For this review, use the dimensioned drawing (mm, ordinates from the lowest corner) and the shaded views. A direction names the side the tool comes from. Give positions to 0.01 mm unless a question says otherwise; leave off trailing zeros. Order: outer loops, then holes, each group sorted by start corner. A loop starts at its lowest first (then second) coordinate and runs counter-clockwise, first axis right, second up. Notation, with made-up numbers: (71.25, -9.5) - (106.25, -9.5) arc R15 ccw to (106.25, 16.5) - close; hole circle Ø8 at (60.5, 21). An arc over 180 degrees is marked (long way). One line per item, written item: value.
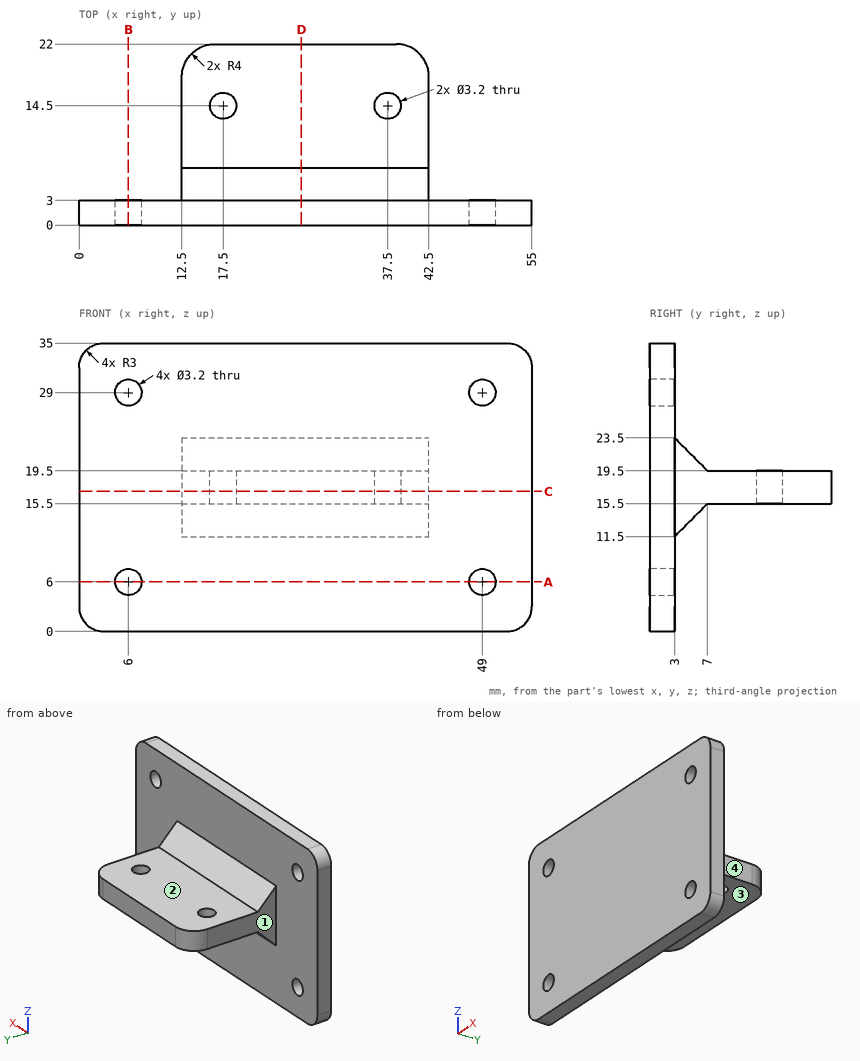
(1) Wall thickness on line 1 (X direction, y = 2.3, z = 29); line 2 (Y direction, x = 17.5, z = 18.65); line 3 (Y direction, x = 5, z = 17.5): over which ranges is each line inside the solid? List them lowest first. Write a range as from..to.
Answers below:
line 1: x = 0..4.4, 7.6..47.4, 50.6..55
line 2: y = 0..12.9, 16.1..22
line 3: y = 0..3
(2) Take a section at B-B (x = 6). Write out the cut boundary in (y, z).
Answers below:
outline: (0, 0) - (3, 0) - (3, 4.4) - (0, 4.4) - close; (0, 7.6) - (3, 7.6) - (3, 27.4) - (0, 27.4) - close; (0, 30.6) - (3, 30.6) - (3, 35) - (0, 35) - close
(3) Machinability: for the marked faces 1, 2, 3 and 4, which of the approach directions +Z, -Z, +X, -X, +Y, -Y give a long, thin tool a straight path to every point of the face, cutting with its end or side? Answer none if there is none.
Answers below:
face 1: +Z, -Z, -X, +Y
face 2: +Z, +X, -X, +Y
face 3: -Z, +X, -X, +Y
face 4: +Z, -Z, +X, +Y
(4) Take a section at A-A (z = 6). Write out the cut boundary in (x, y), then the cut area to 3 significant figures.
Answers below:
outline: (0, 0) - (4.4, 0) - (4.4, 3) - (0, 3) - close; (7.6, 0) - (47.4, 0) - (47.4, 3) - (7.6, 3) - close; (50.6, 0) - (55, 0) - (55, 3) - (50.6, 3) - close
area: 146 mm^2
(5) Take a section at C-C (z = 17). Write out the cut boundary in (x, y), then the cut area to 3 significant figures.
Answers below:
outline: (0, 0) - (55, 0) - (55, 3) - (42.5, 3) - (42.5, 18) arc R4 ccw to (38.5, 22) - (16.5, 22) arc R4 ccw to (12.5, 18) - (12.5, 3) - (0, 3) - close; hole circle Ø3.2 at (17.5, 14.5); hole circle Ø3.2 at (37.5, 14.5)
area: 712 mm^2
(6) For P1, Ø5, axis at x = 37.5, y = 14.5, coming from the -Z side; P2, Ø6, axis at x = 20, y = 11, coming from the +Z side; P3, Ø9.5, axis at y = 9, z = 16.5, coming from the -X side, all flat-tipped, find the tip position at first contact; note any pin that passes through.
Answers below:
P1: stops at z = 15.5
P2: stops at z = 19.5
P3: stops at x = 12.5
(7) Take a section at D-D (x = 27). Write out the cut boundary in (y, z).
Answers below:
outline: (0, 0) - (3, 0) - (3, 11.5) - (7, 15.5) - (22, 15.5) - (22, 19.5) - (7, 19.5) - (3, 23.5) - (3, 35) - (0, 35) - close
